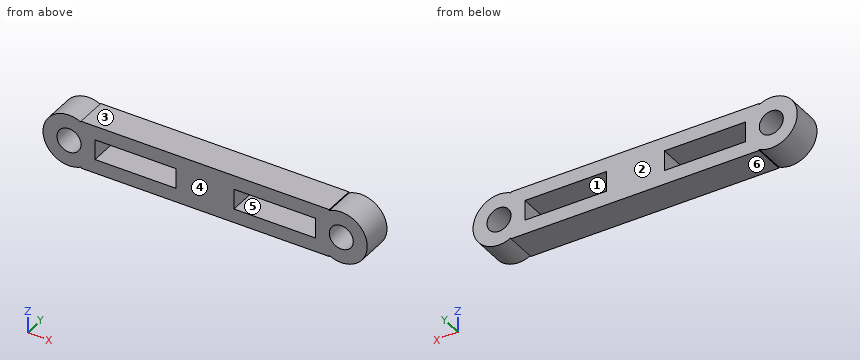
from build123d import *

# Parameters (mm, degrees)
SKETCH1_W                = 22.609360872
SKETCH1_H                = 4.3815
SKETCH1_W_2              = 7.366
SKETCH1_H_2              = 1.8415
SKETCH1_W_3              = 7.407296779
BOSS_EXTRUDE1_DEPTH      = 6.35
BOSS_EXTRUDE2_REACH      = 15.15
BOSS_EXTRUDE3_START      = 2.19075
BOSS_EXTRUDE3_DEPTH      = 2.19075
SKETCH7_R                = 1.5875
BOSS_EXTRUDE4_DEPTH      = 1.27
MIRROR2_COPY_1_SKETCH_R  = 1.5875
MIRROR2_COPY_1_DEPTH     = 1.27
BOSS_EXTRUDE5_DEPTH      = 6.35
BOSS_EXTRUDE5_DEPTH_BACK = 1.27
SKETCH8_R                = 0.635
SKETCH9_W                = 22.609360872
SKETCH9_H                = 6.35
BOSS_EXTRUDE6_DEPTH      = 4.3815
SKETCH10_W               = 6.35
SKETCH10_H               = 1.8415
CUT_EXTRUDE1_DEPTH       = 12.7
CUT_EXTRUDE2_DEPTH       = 23.114
CUT_EXTRUDE2_DEPTH_BACK  = 4.7625
SKETCH12_W               = 31.633822951
SKETCH12_H               = 14.456952732
SKETCH13_W               = 7.366
SKETCH13_H               = 1.8415
SKETCH13_W_2             = 7.407296779
CUT_EXTRUDE3_DEPTH       = 12.7
SKETCH15_W               = 5.299628269
SKETCH15_H               = 4.3815
SKETCH15_W_2             = 5.528427798
CUT_EXTRUDE5_DEPTH       = 2.8575
SKETCH14_R               = 2.367055436
SKETCH14_R_2             = 1.095375
BOSS_EXTRUDE9_DEPTH      = 2.8575


with BuildPart() as part:
    # Sketch1 → Boss-Extrude1 (new body)
    with BuildSketch(Plane(origin=(0, 0, 0), x_dir=(1, 0, 0), z_dir=(0, 1, 0))):
        Rectangle(SKETCH1_W, SKETCH1_H)
        with Locations((-6.35, 0)):
            Rectangle(SKETCH1_W_2, SKETCH1_H_2, mode=Mode.SUBTRACT)
        with Locations((6.329351611, 0)):
            Rectangle(SKETCH1_W_3, SKETCH1_H_2, mode=Mode.SUBTRACT)
    extrude(amount=BOSS_EXTRUDE1_DEPTH)

    # Boss-Extrude2: up to this face of the body (flat: up to its plane)
    boss_extrude2_end = Plane(part.part.faces().sort_by_distance((0, 3.175, -2.19075))[0])
    # Sketch2 → Boss-Extrude2 (add, up to the picked face)
    with BuildSketch(Plane.XY, mode=Mode.PRIVATE) as boss_extrude2_sk1:
        with BuildLine():
            Line((3.175, 0), (-3.175, 0))
            ThreePointArc((-3.175, 0), (0, -3.175), (3.175, 0))
        make_face()
    boss_extrude2_tool1 = split(extrude(boss_extrude2_sk1.sketch, amount=-BOSS_EXTRUDE2_REACH, mode=Mode.PRIVATE), bisect_by=boss_extrude2_end, keep=Keep.BOTH, mode=Mode.PRIVATE)
    add(boss_extrude2_tool1.solids().sort_by(Axis((0, -1.347512, 0), (0, 0, -1)))[0])

    # Sketch2<3> → Boss-Extrude3 (add)
    with BuildSketch(Plane.XY.offset(BOSS_EXTRUDE3_START)):
        with BuildLine():
            Line((3.175, 0), (-3.175, 0))
            ThreePointArc((-3.175, 0), (0, -3.175), (3.175, 0))
        make_face()
    extrude(amount=-BOSS_EXTRUDE3_DEPTH)

    # Sketch7 → Boss-Extrude4 (add)
    with BuildSketch(Plane.XY.offset(2.19075)):
        with BuildLine():
            Line((-9.525, 0), (-11.304680436, 0))
            Line((-11.304680436, 0), (-11.304680436, -12.7))
            ThreePointArc((-11.304680436, -12.7), (-8.266575896, -13.958424104), (-9.525, -10.920319564))
            Line((-9.525, -10.920319564), (-9.525, 0))
        make_face()
        with Locations((-9.525, -12.7)):
            Circle(SKETCH7_R, mode=Mode.SUBTRACT)
    boss_extrude4 = extrude(amount=-BOSS_EXTRUDE4_DEPTH)

    # Mirror1: Boss-Extrude4 across plane
    add(boss_extrude4.mirror(Plane(origin=(0, 0, 0), x_dir=(0, 0, 1), z_dir=(1, 0, 0))))

    # Mirror2: Boss-Extrude4 across plane
    add(boss_extrude4.mirror(Plane.XY))

    # Mirror2 copy 1 sketch → Mirror2 copy 1 (add)
    with BuildSketch(Plane(origin=(0, 0, -2.19075), x_dir=(-1, 0, 0), z_dir=(0, 0, -1))):
        with BuildLine():
            Line((-9.525, 0), (-11.304680436, 0))
            Line((-11.304680436, 0), (-11.304680436, -12.7))
            ThreePointArc((-11.304680436, -12.7), (-8.266575896, -13.958424104), (-9.525, -10.920319564))
            Line((-9.525, -10.920319564), (-9.525, 0))
        make_face()
        with Locations((-9.525, -12.7)):
            Circle(MIRROR2_COPY_1_SKETCH_R, mode=Mode.SUBTRACT)
    extrude(amount=-MIRROR2_COPY_1_DEPTH)

    # Sketch8 → Boss-Extrude5 (add, two sides: drawn at the far end of the back side and taken through both)
    # profile 1 of 2: a face of its own
    with BuildSketch(Plane(origin=(0, 6.35, 0), x_dir=(1, 0, 0), z_dir=(0, 1, 0)).offset(-BOSS_EXTRUDE5_DEPTH_BACK)):
        with BuildLine():
            Line((-11.304680436, 2.19075), (-11.304680436, -2.19075))
            ThreePointArc((-11.304680436, -2.19075), (-13.495430436, 0), (-11.304680436, 2.19075))
        make_face()
        with Locations(Location((-12.400055436, 0, 0), (0, 0, 270))):
            Circle(SKETCH8_R, mode=Mode.SUBTRACT)
    # profile 2 of 2: a face of its own
    with BuildSketch(Plane(origin=(0, 6.35, 0), x_dir=(1, 0, 0), z_dir=(0, 1, 0)).offset(-BOSS_EXTRUDE5_DEPTH_BACK)):
        with BuildLine():
            Line((11.304680436, 2.19075), (11.304680436, -2.19075))
            ThreePointArc((11.304680436, -2.19075), (13.495430436, 0), (11.304680436, 2.19075))
        make_face()
        with Locations(Location((12.400055436, 0, 0), (0, 0, 90))):
            Circle(SKETCH8_R, mode=Mode.SUBTRACT)
    extrude(amount=BOSS_EXTRUDE5_DEPTH + BOSS_EXTRUDE5_DEPTH_BACK)

    # Sketch9 → Boss-Extrude6 (add)
    with BuildSketch(Plane(origin=(0, 0, -2.19075), x_dir=(-1, 0, 0), z_dir=(0, 0, -1))):
        with Locations((0, 9.525)):
            Rectangle(SKETCH9_W, SKETCH9_H)
    extrude(amount=-BOSS_EXTRUDE6_DEPTH)

    # Sketch10 → Cut-Extrude1 (cut)
    with BuildSketch(Plane(origin=(0, 12.7, 0), x_dir=(1, 0, 0), z_dir=(0, 1, 0))):
        with Locations((6.308703221, 0)):
            Rectangle(SKETCH10_W, SKETCH10_H)
        with Locations((-6.35, 0)):
            Rectangle(SKETCH10_W, SKETCH10_H)
    extrude(amount=-CUT_EXTRUDE1_DEPTH, mode=Mode.SUBTRACT)

    # Sketch12 → Cut-Extrude2 (cut, two sides: drawn at the far end of the back side and taken through both)
    with BuildSketch(Plane(origin=(0, 5.08, 0), x_dir=(-1, 0, 0), z_dir=(0, -1, 0)).offset(-CUT_EXTRUDE2_DEPTH_BACK)):
        with Locations((-0.08433307, 1.389523064)):
            Rectangle(SKETCH12_W, SKETCH12_H)
    extrude(amount=CUT_EXTRUDE2_DEPTH + CUT_EXTRUDE2_DEPTH_BACK, mode=Mode.SUBTRACT)

    # Sketch13 → Cut-Extrude3 (cut)
    with BuildSketch(Plane(origin=(0, 0, 0), x_dir=(1, 0, 0), z_dir=(0, 1, 0))):
        with Locations((-6.35, 0)):
            Rectangle(SKETCH13_W, SKETCH13_H)
        with Locations((6.329351611, 0)):
            Rectangle(SKETCH13_W_2, SKETCH13_H)
    extrude(amount=CUT_EXTRUDE3_DEPTH, mode=Mode.SUBTRACT)

    # Sketch15 → Cut-Extrude5 (cut)
    with BuildSketch(Plane(origin=(0, 12.7, 0), x_dir=(1, 0, 0), z_dir=(0, 1, 0))):
        with Locations((-13.95449457, 0)):
            Rectangle(SKETCH15_W, SKETCH15_H)
        with Locations((14.068894335, 0)):
            Rectangle(SKETCH15_W_2, SKETCH15_H)
    extrude(amount=-CUT_EXTRUDE5_DEPTH, mode=Mode.SUBTRACT)

    # Sketch14 → Boss-Extrude9 (add)
    # profile 1 of 2: a face of its own
    with BuildSketch(Plane(origin=(0, 12.7, 0), x_dir=(1, 0, 0), z_dir=(0, 1, 0))):
        with Locations((-12.400055436, 0)):
            Circle(SKETCH14_R)
        with Locations(Location((-12.400055436, 0, 0), (0, 0, 270))):
            Circle(SKETCH14_R_2, mode=Mode.SUBTRACT)
    # profile 2 of 2: a face of its own
    with BuildSketch(Plane(origin=(0, 12.7, 0), x_dir=(1, 0, 0), z_dir=(0, 1, 0))):
        with Locations((12.400055436, 0)):
            Circle(SKETCH14_R)
        with Locations(Location((12.400055436, 0, 0), (0, 0, 270))):
            Circle(SKETCH14_R_2, mode=Mode.SUBTRACT)
    extrude(amount=-BOSS_EXTRUDE9_DEPTH)


solid = part.part
Geometry: final body of the model. Coordinates: model frame, mm. Face numbers are marked on the shaded views. A direction names the side the tool comes from. Give positions to 0.01 mm unless a question says otherwise; leave off trailing zeros. Order: outer loops, then holes, each group sorted by start corner. A loop starts at its lowest first (then second) coordinate and runs counter-clockwise, first axis right, second up. Notation, with made-up numbers: (77.5, 59.25) -> (118.5, 59.25) arc R10 cw to (118.5, 72.25) -> close; hole circle Ø11 at (78.5, 21.5). An arc over 180 degrees is marked (long way). Answer as a JSON object with one key per item and string values.
Q1. Section A-A (x = 8). Output: boundary loops of the cut face in (y, z).
Entries:
{"outline": "(9.84, -2.19) -> (12.7, -2.19) -> (12.7, -0.92) -> (9.84, -0.92) -> close; (9.84, 0.92) -> (12.7, 0.92) -> (12.7, 2.19) -> (9.84, 2.19) -> close"}
Q2. Section C-C (y = 10.95). Output: boundary loops of the cut face in (x, z), plus the area to 3 significant figures.
Entries:
{"outline": "(-11.3, -2.19) -> (11.3, -2.19) -> (11.3, -2.1) arc R2.37 ccw (long way) to (11.3, 2.1) -> (11.3, 2.19) -> (-11.3, 2.19) -> (-11.3, 2.1) arc R2.37 ccw (long way) to (-11.3, -2.1) -> close; hole circle Ø2.19 at (-12.4, 0); hole (-10.03, -0.92) -> (-2.67, -0.92) -> (-2.67, 0.92) -> (-10.03, 0.92) -> close; hole (2.63, -0.92) -> (10.03, -0.92) -> (10.03, 0.92) -> (2.63, 0.92) -> close; hole circle Ø2.19 at (12.4, 0)", "area": "91.9 mm^2"}
Q3. Material intervals for probe 1 along X at (y, z) = (11.15, 0); probe 2 along Z at (x, y) = (-9.25, 11.05); probe 3 along Z at (x, y) = (-11.25, 11.65), sorted ascending.
Entries:
{"probe 1": "x = -14.77 to -13.5, -11.3 to -10.03, -2.67 to 2.63, 10.03 to 11.3, 13.5 to 14.77", "probe 2": "z = -2.19 to -0.92, 0.92 to 2.19", "probe 3": "z = -2.19 to 2.19"}
Q4. First-contact query: pin 1 (0.9 mm diameter, centred on x = 7.5, y = 10.5, fed in from -Z); pin 2 (0.9 mm diameter, centred on y = 11.5, z = -0.5, fed in from -X); pin 3 (1.5 mm diameter, centred on x = -11, y = 11.5, fed in from -Z). Flat tips, straight axial feed; report the tip coordinate or a pass-through.
Entries:
{"pin 1": "stops at z = -2.19", "pin 2": "stops at x = -14.77", "pin 3": "stops at z = -2.28"}
Q5. Section D-D (z = -1.8). Output: boundary loops of the cut face in (x, y), plus the area to 3 significant figures.
Entries:
{"outline": "(-13.94, 9.84) -> (13.94, 9.84) -> (13.94, 12.7) -> (-13.94, 12.7) -> close", "area": "79.7 mm^2"}
Q6. Access query for the marked faces 1 and 2. Directions: +Z, -Z, +X, -X, +Y, -Y. A direction counts if a zero-diameter tool reaches every point of the face in a straight line with its end or side. Return the directions, or none.
Entries:
{"face 1": "+Y, -Y", "face 2": "+Z, -Z, +X, -X, +Y"}
Q7. Section B-B (z = 0). Output: boundary loops of the cut face in (x, y).
Entries:
{"outline": "(-14.77, 9.84) -> (-13.5, 9.84) -> (-13.5, 12.7) -> (-14.77, 12.7) -> close; (-11.3, 9.84) -> (-10.03, 9.84) -> (-10.03, 12.7) -> (-11.3, 12.7) -> close; (-2.67, 9.84) -> (2.63, 9.84) -> (2.63, 12.7) -> (-2.67, 12.7) -> close; (10.03, 9.84) -> (11.3, 9.84) -> (11.3, 12.7) -> (10.03, 12.7) -> close; (13.5, 9.84) -> (14.77, 9.84) -> (14.77, 12.7) -> (13.5, 12.7) -> close"}
Q8. Draft query along Z for the marked faces 3, 4, 5 and 6. Return one class per face: released by +Z, released by -Z, zero draft, split by the parting line, or undercut.
Entries:
{"face 3": "released by +Z", "face 4": "zero draft", "face 5": "undercut", "face 6": "released by -Z"}
